from build123d import *

# Parameters (mm, degrees)
FIXEDMOTOR_R        = 6.207042780583919
FIXEDMOTOR_R_2      = 2.0000000000000004
FIXEDMOTOR_R_3      = 2
FIXEDMOTOR_R_4      = 1.9999999999999996
FIXEDMOTOR_R_5      = 2.0000000000000013
BOSS_EXTRUDE1_DEPTH = 3
BOSS_EXTRUDE2_DEPTH = 3
FILLET2_R           = 1
FILLET3_R           = 2
FILLET4_R           = 1
FILLET5_R           = 1
CUT_EXTRUDE1_DEPTH  = 40
BOSS_EXTRUDE3_DEPTH = 3
CUT_EXTRUDE2_DEPTH  = 40
FILLET6_R           = 2
FILLET7_R           = 1
BOSS_EXTRUDE4_DEPTH = 3
FILLET8_R           = 2
FILLET9_R           = 1
SKETCH9_R           = 2.000000000000003
SKETCH9_R_2         = 2.0000000000000027
CUT_EXTRUDE3_DEPTH  = 3
FILLET10_R          = 2
FILLET11_R          = 2
FILLET15_R          = 1
SKETCH11_R          = 1.9999999999999962
CUT_EXTRUDE4_DEPTH  = 3


with BuildPart() as part:
    # FixedMotor → Boss-Extrude1 (new body)
    with BuildSketch(Plane.XY):
        Polygon((19.000000000955392, 19.999999999092385), (18.99999999904462, -20.000000000907605), (-23.000000000955385, -19.999999998901302), (-23, 1.09869677e-09), (-22.99999999904461, 20.000000001098698), align=None)
        with Locations((-6.884060715651985, 3.2884703e-10)):
            Circle(FIXEDMOTOR_R, mode=Mode.SUBTRACT)
        with Locations((-1.0290674932644954, -15.465801631157241)):
            Circle(FIXEDMOTOR_R_2, mode=Mode.SUBTRACT)
        with Locations((-12.879243355840744, 8.624099406954452)):
            Circle(FIXEDMOTOR_R_3, mode=Mode.SUBTRACT)
        with Locations((13.908310849105225, 6.841702224202803)):
            Circle(FIXEDMOTOR_R_4, mode=Mode.SUBTRACT)
        with Locations((1.0290674932644954, 15.465801631157241)):
            Circle(FIXEDMOTOR_R_5, mode=Mode.SUBTRACT)
    extrude(amount=BOSS_EXTRUDE1_DEPTH)

    # Sketch2 → Boss-Extrude2 (add)
    with BuildSketch(Plane(origin=(19.000000000000007, -9.0761747e-10, 0), x_dir=(0, 0, -1), z_dir=(1.0, -4.776925383032094e-11, 0))):
        Polygon((0, 20), (70, 20), (70, -19.999999999999993), (0, -19.99999999999999), (-3, -19.99999999999999), (-3, 20), align=None)
    extrude(amount=BOSS_EXTRUDE2_DEPTH)

    # Fillet2
    fillet2_edges = [part.edges().sort_by_distance(p)[0] for p in [
        (19.000000000000007, -9.0760821e-10, 0),
    ]]
    fillet(fillet2_edges, radius=FILLET2_R)

    # Fillet3
    fillet3_edges = [part.edges().sort_by_distance(p)[0] for p in [
        (22.000000000000007, -1.05092168e-09, 3),
    ]]
    fillet(fillet3_edges, radius=FILLET3_R)

    # Fillet4
    fillet4_edges = [part.edges().sort_by_distance(p)[0] for p in [
        (-23, 1.09869802e-09, 3),
    ]]
    fillet(fillet4_edges, radius=FILLET4_R)

    # Fillet5
    fillet5_edges = [part.edges().sort_by_distance(p)[0] for p in [
        (-23, 1.09869802e-09, 0),
    ]]
    fillet(fillet5_edges, radius=FILLET5_R)

    # Sketch5 → Cut-Extrude1 (cut)
    with BuildSketch(Plane.XZ.offset(19.999999999999993)):
        Polygon((22.000000000000004, -70), (19.000000000000004, -67), (19.000000000000004, -70), align=None)
    extrude(amount=-CUT_EXTRUDE1_DEPTH, mode=Mode.SUBTRACT)

    # Sketch6 → Boss-Extrude3 (add)
    with BuildSketch(Plane(origin=(-23.99999999999999, 1.14645595e-09, -23.999999999999964), x_dir=(-0.7071067811865471, 3.377778224099027e-11, 0.7071067811865479), z_dir=(-0.7071067811865479, 3.3777782240990306e-11, -0.7071067811865471))):
        Polygon((-65.05382386916239, -19.999999999999993), (-65.05382386916239, 20.000000000000007), (-100.8111831820431, 20.000000000000007), (-100.8111831820431, -20.000000000000004), align=None)
        Polygon((-65.05382386916239, 20.00000000000001), (-65.05382386916239, -19.99999999999999), (-60.81118318204311, -20), (-60.81118318204311, 20.000000000000007), align=None)
    extrude(amount=BOSS_EXTRUDE3_DEPTH)

    # Sketch7 → Cut-Extrude2 (cut)
    with BuildSketch(Plane(origin=(9.5538656e-10, 20.000000000000004, 0), x_dir=(1.0, -4.776932817561277e-11, 0), z_dir=(4.776932817561277e-11, 1.0, 0))):
        Polygon((18.999999999999996, 67), (18.999999999999996, 71.2426406871193), (16.878679656440344, 69.12132034355965), align=None)
    extrude(amount=-CUT_EXTRUDE2_DEPTH, mode=Mode.SUBTRACT)

    # Fillet6
    fillet6_edges = [part.edges().sort_by_distance(p)[0] for p in [
        (18.999999999999996, -9.0761532e-10, -71.2426406871193),
    ]]
    fillet(fillet6_edges, radius=FILLET6_R)

    # Fillet7
    fillet7_edges = [part.edges().sort_by_distance(p)[0] for p in [
        (22.000000000000007, -1.05092168e-09, -70),
    ]]
    fillet(fillet7_edges, radius=FILLET7_R)

    # Sketch8 → Boss-Extrude4 (add)
    with BuildSketch(Plane(origin=(71.28427124746187, -3.40515935e-09, -71.28427124746194), x_dir=(-0.7071067811865479, -3.3777595325221335e-11, -0.7071067811865471), z_dir=(0.7071067811865471, -3.377759532522137e-11, -0.7071067811865479))):
        Polygon((33.94112549560315, 20.0000000022929), (63.94112549560316, 20.0000000022929), (63.94112549560316, -19.99999999770711), (33.94112549830536, -19.99999999770711), align=None)
    extrude(amount=BOSS_EXTRUDE4_DEPTH)

    # Fillet8
    fillet8_edges = [part.edges().sort_by_distance(p)[0] for p in [
        (49.40559159102152, -2.3600452e-09, -97.40559159102156),
    ]]
    fillet(fillet8_edges, radius=FILLET8_R)

    # Fillet9
    fillet9_edges = [part.edges().sort_by_distance(p)[0] for p in [
        (45.16295090390224, -2.15738535e-09, -97.40559159102155),
    ]]
    fillet(fillet9_edges, radius=FILLET9_R)

    # Sketch9 → Cut-Extrude3 (cut)
    with BuildSketch(Plane(origin=(73.40559159102153, -3.50649214e-09, -73.4055915910216), x_dir=(-0.7071067811865479, -3.3777840652168006e-11, -0.7071067811865472), z_dir=(0.7071067811865472, -3.377784065216806e-11, -0.7071067811865479))):
        with Locations((53.94112549560317, 0)):
            Circle(SKETCH9_R)
        with Locations((43.94112549560317, 10)):
            Circle(SKETCH9_R_2)
        with Locations((43.94112549560317, -10)):
            Circle(SKETCH9_R_2)
    extrude(amount=-CUT_EXTRUDE3_DEPTH, mode=Mode.SUBTRACT)

    # Fillet10
    fillet10_edges = [part.edges().sort_by_distance(p)[0] for p in [
        (27.131727984600627, 19.9999999966773, -117.55813485483814),
    ]]
    fillet(fillet10_edges, radius=FILLET10_R)

    # Fillet11
    fillet11_edges = [part.edges().sort_by_distance(p)[0] for p in [
        (27.131727984600627, -20.00000000332271, -117.55813485292741),
    ]]
    fillet(fillet11_edges, radius=FILLET11_R)

    # Fillet15
    fillet15_edges = [part.edges().sort_by_distance(p)[0] for p in [
        (32.02081528112668, 19.999999998470404, -84.2634559672906),
        (32.02081527921592, -20.000000001529603, -84.2634559672906),
        (19.00000000095539, 19.99999999909238, -35.70710678118655),
        (19.15224093593281, 19.999999999085112, -71.17958042710328),
        (19.152240934022036, -20.000000000914874, -71.17958042710328),
        (22.000000000955392, 19.999999998949075, -34.292893218813454),
        (34.78858223218229, -20.000000001661814, -82.78858223313767),
        (34.788582234093056, 19.999999998338193, -82.78858223313767),
        (22.076120468444106, 19.99999999894544, -69.96846986999199),
        (22.076120466533336, -20.00000000105455, -69.968469869992),
        (38.79898987322329, -20.000000002866717, -108.01219330786441),
        (48.57716446531997, -20.00000000245559, -97.40559159102156),
        (48.577164467230716, 19.999999997544418, -97.40559159102156),
        (35.9705627484771, -20.000000002799162, -106.5979797454913),
        (44.74873734248451, 19.999999997862385, -97.40559159102156),
        (44.74873734057375, -20.0000000021376, -97.40559159102156),
        (38.79898987417868, 19.999999997133294, -108.01219330881977),
        (35.970562749432474, 19.99999999720085, -106.59797974644667),
        (26.485281375193907, 19.414213559120846, -116.08326112065726),
        (28.60660171875356, 19.414213559019515, -118.20458146421691),
        (26.071067812820807, -3.27204382e-09, -116.49747468210296),
        (28.192388156380453, -3.37337661e-09, -118.6187950256626),
        (26.485281375193892, -19.41421356562536, -116.08326111880247),
        (28.606601718753545, -19.41421356572669, -118.20458146236213),
        (18.999999999044615, -20.00000000090761, -35.70710678118655),
        (18.707106780231165, -20.000000000893618, -0.2928932188134521),
        (18.70710678214194, 19.999999999106375, -0.2928932188134509),
        (21.999999999044622, -20.000000001050918, -34.292893218813454),
        (21.414213561417718, -20.00000000102293, 2.414213562373094),
        (21.414213563328484, 19.999999998977056, 2.4142135623730967),
        (-23.000000000955385, -19.999999998901302, 1.5),
        (-22.99999999904461, 20.000000001098698, 1.5),
        (-0.9999999990446042, 20.00000000004777, 3),
        (-22.707106780231157, 20.000000001084707, 2.7071067811865466),
        (-1.0000000009553816, -19.999999999952223, 3),
        (-22.707106782141928, -19.999999998915293, 2.707106781186548),
        (-1.9999999990446113, 20.00000000009554, 0),
        (-2.000000000955385, -19.999999999904453, 0),
        (-22.707106780231157, 20.000000001084707, 0.2928932188134523),
        (-22.707106782141935, -19.999999998915293, 0.29289321881345365),
    ]]
    fillet(fillet15_edges, radius=FILLET15_R)

    # Sketch11 → Cut-Extrude4 (cut)
    with BuildSketch(Plane(origin=(-26.121320343559653, 1.24778636e-09, -26.121320343559624), x_dir=(-0.7071067811865472, 3.377767510137627e-11, 0.7071067811865478), z_dir=(-0.7071067811865478, 3.37776751013763e-11, -0.7071067811865472))):
        with Locations((-92.81118318204305, 10)):
            Circle(SKETCH11_R)
        with Locations((-92.81118318204305, -10)):
            Circle(SKETCH11_R)
    extrude(amount=-CUT_EXTRUDE4_DEPTH, mode=Mode.SUBTRACT)


solid = part.part
Geometry: final body of the model. Coordinates: model frame, mm. A direction names the side the tool comes from. Give positions to 0.01 mm unless a question says otherwise; leave off trailing zeros. Order: outer loops, then holes, each group sorted by start corner. A loop starts at its lowest first (then second) coordinate and runs counter-clockwise, first axis right, second up. Notation, with made-up numbers: (63, -21) -> (96, -21) arc R22 cw to (96, 10) -> close; hole circle Ø9 at (-31.5, 63.5). An arc over 180 degrees is marked (long way). Write each question's results on one line, items separated by ' | '.
1) Set-up query: faces 4 (the face through (32.059, -19.715, -83.877)), 5 (the face through (22, 0, -35)), 6 (the face through (32.408, 19.715, -84.225)). Return all of +Z, -Z, +X, -X, +Y, -Y with unobstructed straight access to the full face (end or side cutting, diameter ignored); none if empty.
Geometry says:
face 4: -X, -Y | face 5: +Z, +X, +Y, -Y | face 6: -X, +Y
2) Line query: line 1 along Z through (x, y) = (-19, -16.5); line 2 along X through (y, z) = (0, -48.5); line 3 along Z through (x, y) = (44, -13.5). Output: solid intervals per line, ascending.
Geometry says:
line 1: z = 0 to 3 | line 2: x = 19 to 22 | line 3: z = -102.81 to -98.57, -96.24 to -92
3) Cut plane C-C (y = 0). Output: boundary loops of the cut face in (x, z).
Geometry says:
outline: (-23, 1) arc R1 ccw to (-22, 0) -> (-13.09, 0) -> (-13.09, 3) -> (-22, 3) arc R1 ccw to (-23, 2) -> close; (-0.68, 0) -> (18, 0) arc R1 cw to (19, -1) -> (19, -70.41) arc R2 ccw to (19.59, -71.83) -> (44.46, -96.7) arc R1 cw to (44.46, -98.11) -> (34.56, -108.01) -> (36.68, -110.13) -> (47.99, -98.82) arc R2 ccw to (47.99, -95.99) -> (22.29, -70.29) arc R1 cw to (22, -69.59) -> (22, 1) arc R2 ccw to (20, 3) -> (-0.68, 3) -> close; (26.78, -117.2) -> (27.49, -117.91) arc R1 ccw to (28.9, -117.91) -> (33.85, -112.96) -> (31.73, -110.84) -> (26.78, -115.79) arc R1 ccw to start
4) Cut plane B-B (x = 14). Output: boundary loops of the cut face in (y, z).
Geometry says:
outline: (-20, 1) arc R1 ccw to (-19, 0) -> (4.84, 0) -> (4.84, 3) -> (-19, 3) arc R1 ccw to (-20, 2) -> close; (8.84, 0) -> (19, 0) arc R1 ccw to (20, 1) -> (20, 2) arc R1 ccw to (19, 3) -> (8.84, 3) -> close
5) Cut plane A-A (z = -43.5). Output: boundary loops of the cut face in (x, y), and give its area (3 significant figures).
Geometry says:
outline: (19, -19) arc R1 ccw to (20, -20) -> (21, -20) arc R1 ccw to (22, -19) -> (22, 19) arc R1 ccw to (21, 20) -> (20, 20) arc R1 ccw to (19, 19) -> close | area: 119 mm²
6) Cut plane D-D (x = 4.5). Output: boundary loops of the cut face in (y, z).
Geometry says:
outline: (-20, 1) arc R1 ccw to (-19, 0) -> (19, 0) arc R1 ccw to (20, 1) -> (20, 2) arc R1 ccw to (19, 3) -> (-19, 3) arc R1 ccw to (-20, 2) -> close
7) First-contact query: pin 1 Ø5 at (x, y) = (-12.88, 8.62) entering from -Z; pin 2 Ø8 at (y, z) = (9, -85) entering from -X; pin 3 Ø12 at (y, z) = (-4.5, -78.5) entering from +X. Flat tips, straight axial feed; report the tip coordinate or a pass-through.
Geometry says:
pin 1: stops at z = 0 | pin 2: stops at x = 28.76 | pin 3: stops at x = 36.5
8) Draft query along X for faces 1 (the face through (2.104, 17.152, 1.479)), 2 (the face through (3, 0, 0)), 3 (the face through (19, 0, -36)). Return one class per face: released by +X, released by -X, zero draft, split by the parting line, or undercut.
Geometry says:
face 1: undercut | face 2: zero draft | face 3: released by -X
